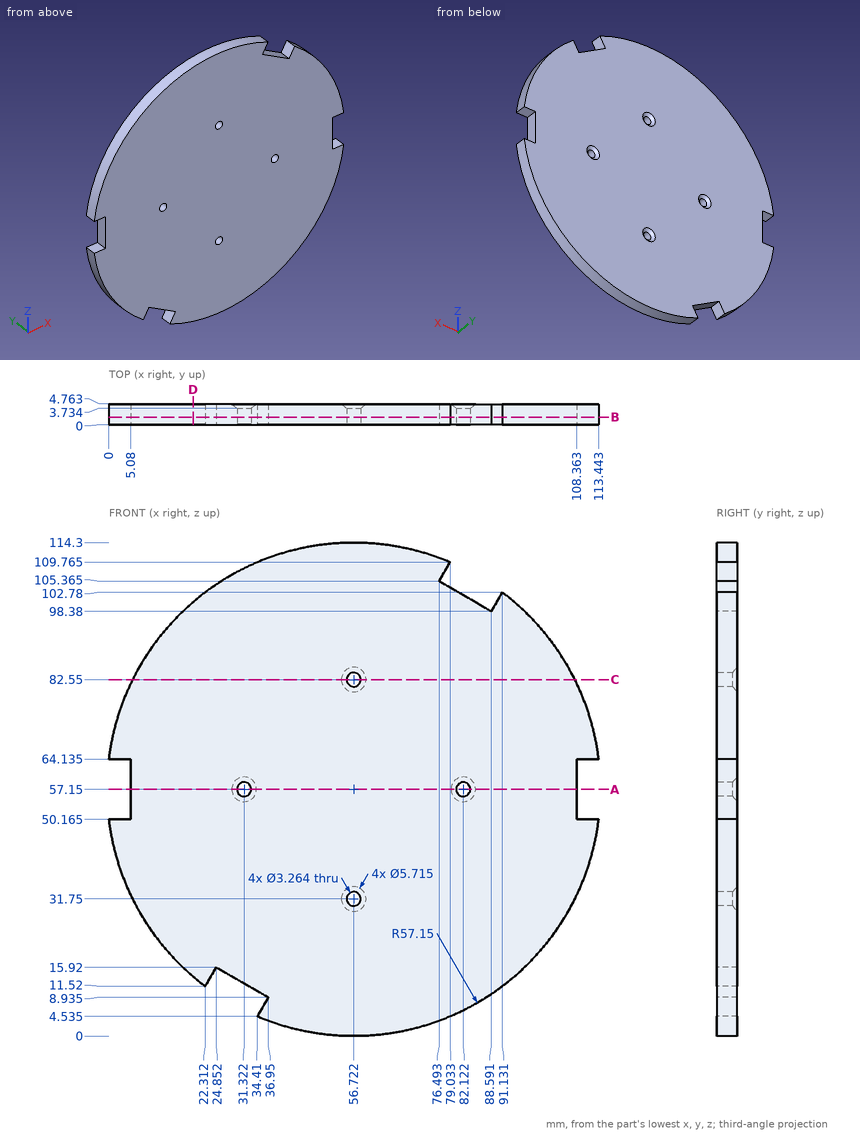
Check sheet for the drawn part. Datum: minimum x, y, z corner. Units: mm. Round coordinates to 2 decimals unless told otherwise and drop trailing zeros. Loops run counter-clockwise (first coordinate to the right, second up) from the corner with the lowest first, then second, coordinate; pieces in that order, holes last. Notation, with made-up numbers: (-9.5, -30.75) - (46.5, -30.75) arc R14 ccw to (46.5, -9.75) - close; hole circle Ø10 at (82, 71). An arc over 180 degrees is marked (long way). Write each question's results on one line, items separated by ' | '. Start each with the question number.
Q1. Gauge pin test, flat ends, axial feed: P1, Ø2, axis at x = 15, y = 0.5, coming from the +Z side; P2, Ø5, axis at x = 82.12, z = 57.15, coming from the +Y side (1 decimal); P3, Ø2.5, axis at y = 3.5, z = 57.5, coming from the +X side. Record the tip position at first contact, or that the pin passes through.
Q2. Cross-section at A-A on z = 57.15. Enter the section's corners in (x, y) (1 decimal), and give its area (3 significant figures).
Q3. Cross-section at C-C on z = 82.55. Enter the section's corners in (x, y) (1 decimal), and give its area (3 significant figures).
Q4. Cross-section at D-D on x = 19.5. Enter the section's corners in (y, z).
Q5. Thickness scan on line 1 (X direction, y = 1.6, z = 57.15); line 2 (X direction, y = 1.8, z = 31.75) (1 decimal); line 3 (Z direction, x = 78, y = 2.05) (1 decimal). Record the ranges inside material, lowest first. Write a range as [from, to].
Q6. Cross-section at B-B on y = 1.7. State how many separate pieces and enclosed holes the cut face has, and give its area (3 significant figures).
Answers below:
1) P1: stops at z = 97.25 | P2: stops at y = 4.5 | P3: stops at x = 108.36
2) outline: (5.1, 0) - (29.7, 0) - (29.7, 3.7) - (28.5, 4.8) - (5.1, 4.8) - close; (33, 0) - (80.5, 0) - (80.5, 3.7) - (79.3, 4.8) - (34.2, 4.8) - (33, 3.7) - close; (83.8, 0) - (108.4, 0) - (108.4, 4.8) - (85, 4.8) - (83.8, 3.7) - close | area: 458 mm²
3) outline: (5.5, 0) - (55.1, 0) - (55.1, 3.7) - (53.9, 4.8) - (5.5, 4.8) - close; (58.4, 0) - (107.9, 0) - (107.9, 4.8) - (59.6, 4.8) - (58.4, 3.7) - close | area: 471 mm²
4) outline: (0, 13.78) - (4.76, 13.78) - (4.76, 100.52) - (0, 100.52) - close
5) line 1: x = [5.08, 29.69], [32.95, 80.49], [83.75, 108.36] | line 2: x = [5.5, 55.1], [58.4, 107.9] | line 3: z = [4.1, 104.5], [108, 110.2]
6) separate pieces: 1 | enclosed holes: 4 | area: 9,930 mm²
